Geometry: final body of the model. Coordinates: model frame, mm. A direction names the side the tool comes from. Round coordinates to 2 decimals unless told otherwise and drop trailing zeros. Order: outer loops, then holes, each group sorted by start corner. A loop starts at its lowest first (then second) coordinate and runs counter-clockwise, first axis right, second up. Notation, with made-up numbers: M 52,75 L 107,75 A27 ccw 107,102 Z; hole C 88.5,22 d10. An arc over 180 degrees is marked long. Put each result on its own line as item: value. Start each with the question number.
1) Access query for faces 4 (the flat face through (-25.4, 0.2, 7)), 5 (the flat face through (0, 0, 7)). Directions: +Z, -Z, +X, -X, +Y, -Y. A direction counts if a zero-diameter tool reaches every point of the face in a straight line with its end or side. Return the directions, or none.
2) Material intervals for probe 1 along X at (y, z) = (1.25, -2.54); probe 2 along Y at (x, z) = (21, -9); probe 3 along Z at (x, y) = (-7, 0.45), sorted ascending. Write a range as [from, to].
3) Section B-B, the plane z = -2.54. Return loops of the section in (x, y).
4) First-contact query: P1, Ø2, axis at x = -10, y = 0.5, coming from the +Z side; P2, Ø12, axis at x = 8.5, z = 12, coming from the -Y side; P3, Ø2, axis at y = 0.5, z = -11, coming from the +X side. Flat tips, straight axial feed; report the tip coordinate or a pass-through.
5) Draft query along Z for faces 1 (the flat face through (-0.36, -1.94, 18.6)), 2 (the cylindrical face through (-8.69, 0.75, -1.4)), 3 (the flat face through (-0.36, -3.19, 22.49)). Return one class per face: pulls with the +Z half, pulls with the -Z half, needs draft (parallel to the pull), parting line crosses it, or undercut.
6) Section A-A, the plane x = 0. Return loops of the section in (y, z), then the cut area to 3 significant figures.
7) Section C-C, the plane x = -13. Return loops of the section in (y, z).
8) Section D-D, the plane x = -6. Return loops of the section in (y, z).
from build123d import *

# Parameters (mm, degrees)
SKETCH1_W           = 50.8
SKETCH1_H           = 30.48
SKETCH1_R           = 8.763
BOSS_EXTRUDE1_DEPTH = 1.524
BOSS_EXTRUDE2_DEPTH = 50.8
FILLET1_R           = 6.35


with BuildPart() as part:
    # Sketch1 → Boss-Extrude1 (new body)
    with BuildSketch(Plane(origin=(0, 0, 0), x_dir=(1, 0, 0), z_dir=(0, 1, 0))):
        Rectangle(SKETCH1_W, SKETCH1_H)
        with Locations(Location((0, 2.54, 0), (0, 0, 90))):
            Circle(SKETCH1_R, mode=Mode.SUBTRACT)
    extrude(amount=BOSS_EXTRUDE1_DEPTH)

    # Sketch2 → Boss-Extrude2 (add)
    with BuildSketch(Plane.ZY.offset(25.4)):
        Polygon((15.24, 0), (22.059084029, -3.937), (22.93896584, -2.413), (16.11988181, 1.524), (15.24, 1.524), align=None)
    extrude(amount=-BOSS_EXTRUDE2_DEPTH)

    # Fillet1
    fillet1_edges = [part.edges().sort_by_distance(p)[0] for p in [
        (0, 1.524, 16.11988181),
        (-25.4, 0.762, -15.24),
        (25.4, 0.762, -15.24),
    ]]
    fillet(fillet1_edges, radius=FILLET1_R)


solid = part.part
Result sheet:
1. face 4: +Z, -Z, -X, +Y, -Y
1. face 5: -Z, +X, -X, -Y
2. probe 1: x = [-25.4, -8.76], [8.76, 25.4]
2. probe 2: y = [0, 1.52]
2. probe 3: z = [-15.24, -7.81], [2.73, 17.98]
3. outline: M -25.4,0 L -8.76,0 L -8.76,1.52 L -25.4,1.52 Z; M 8.76,0 L 25.4,0 L 25.4,1.52 L 8.76,1.52 Z
4. P1: stops at z = 19.63
4. P2: stops at y = -1.59
4. P3: stops at x = 25.3
5. face 1: pulls with the -Z half
5. face 2: undercut
5. face 3: pulls with the +Z half
6. outline: M -3.94,22.06 L 0,15.24 L 0,6.22 L 1.52,6.22 L 1.52,14.42 A6.35 ccw 0.67,17.59 L -2.41,22.94 Z; M 0,-15.24 L 1.52,-15.24 L 1.52,-11.3 L 0,-11.3 Z
6. area: 34.0 mm2
7. outline: M -3.94,22.06 L 0,15.24 L 0,-15.24 L 1.52,-15.24 L 1.52,14.42 A6.35 ccw 0.67,17.59 L -2.41,22.94 Z
8. outline: M -3.94,22.06 L 0,15.24 L 0,3.85 L 1.52,3.85 L 1.52,14.42 A6.35 ccw 0.67,17.59 L -2.41,22.94 Z; M 0,-15.24 L 1.52,-15.24 L 1.52,-8.93 L 0,-8.93 Z
